```python
from build123d import *
from build123d import SkipClean  # not in build123d's __all__

# Parameters (mm, degrees)
F0_W      = 40
F0_H      = 30
F1_DEPTH  = 52
F2_R      = 5
F3_DEPTH  = 20
F4_R      = 1.65
F5_DEPTH  = 10
F6_R      = 2.5
F7_DEPTH  = 52.001
F8_R      = 4
F9_DEPTH  = 5
F10_W     = 40
F10_H     = 35
F11_DEPTH = 10
F12_W     = 40
F12_H     = 35
F13_DEPTH = 10
F15_DEPTH = 5
F16_R     = 2.15
F17_DEPTH = 40.001
F18_R     = 5
F19_DEPTH = 40.001
F20_R     = 6
F21_DEPTH = 1
F22_R     = 2.25
F23_DEPTH = 15.5358573251


with BuildPart() as f1:
    # F0 (on Top) → F1 (new body)
    with BuildSketch(Plane.XY):
        with Locations((20, 15)):
            Rectangle(F0_W, F0_H)
    extrude(amount=F1_DEPTH)

    # F2 (on face) → F3 (cut)
    with BuildSketch(Plane.XZ):
        with Locations((20, 42)):
            Circle(F2_R)
    extrude(amount=-F3_DEPTH, mode=Mode.SUBTRACT)

    # F4 (on face) → F5 (cut)
    with BuildSketch(Plane.XY.offset(52)):
        with Locations((20, 5)):
            Circle(F4_R)
        with Locations((20, 25)):
            Circle(F4_R)
    extrude(amount=-F5_DEPTH, mode=Mode.SUBTRACT)

    # F6 (on face) → F7 (cut, through all)
    with BuildSketch(Plane.XY.offset(52)):
        with Locations((5, 5)):
            Circle(F6_R)
        with Locations((5, 25)):
            Circle(F6_R)
        with Locations((35, 5)):
            Circle(F6_R)
        with Locations((35, 25)):
            Circle(F6_R)
    extrude(amount=-F7_DEPTH, mode=Mode.SUBTRACT)

    # F8 (on face) → F9 (cut)
    with BuildSketch(Plane.XY.offset(52)):
        with Locations((5, 25)):
            Circle(F8_R)
        with Locations((5, 5)):
            Circle(F8_R)
        with Locations((35, 25)):
            Circle(F8_R)
        with Locations((35, 5)):
            Circle(F8_R)
    extrude(amount=-F9_DEPTH, mode=Mode.SUBTRACT)

    # F10 (on face) → F11 (join)
    with BuildSketch(Plane.XZ):
        with Locations((20, 17.5)):
            Rectangle(F10_W, F10_H)
    extrude(amount=F11_DEPTH)

    # F12 (on face) → F13 (join)
    with BuildSketch(Plane(origin=(0, 30, 0), x_dir=(-1, 0, 0), z_dir=(0, 1, 0))):
        with Locations((-20, 17.5)):
            Rectangle(F12_W, F12_H)
    extrude(amount=F13_DEPTH)

    # F14 (on face) → F15 (cut)
    with BuildSketch(Plane.XY.offset(35)):
        with BuildLine():
            Line((6.5, 31), (33.5, 31))
            ThreePointArc((33.5, 31), (36.3284271247, 32.1715728753), (37.5, 35))
            ThreePointArc((37.5, 35), (36.3284271247, 37.8284271247), (33.5, 39))
            Line((33.5, 39), (6.5, 39))
            ThreePointArc((6.5, 39), (3.6715728753, 37.8284271247), (2.5, 35))
            ThreePointArc((2.5, 35), (3.6715728753, 32.1715728753), (6.5, 31))
        make_face()
        with BuildLine():
            Line((6.5, -9), (33.5, -9))
            ThreePointArc((33.5, -9), (36.3284271247, -7.8284271247), (37.5, -5))
            ThreePointArc((37.5, -5), (36.3284271247, -2.1715728753), (33.5, -1))
            Line((33.5, -1), (6.5, -1))
            ThreePointArc((6.5, -1), (3.6715728753, -2.1715728753), (2.5, -5))
            ThreePointArc((2.5, -5), (3.6715728753, -7.8284271247), (6.5, -9))
        make_face()
    extrude(amount=-F15_DEPTH, mode=Mode.SUBTRACT)

    # F16 (on face) → F17 (cut, through all)
    with BuildSketch(Plane(origin=(0, 0, 0), x_dir=(0, -1, 0), z_dir=(-1, 0, 0))):
        with Locations((-15, 32)):
            Circle(F16_R)
        with Locations((-35, 32)):
            Circle(F16_R)
        with Locations((5, 32)):
            Circle(F16_R)
    extrude(amount=-F17_DEPTH, mode=Mode.SUBTRACT)

    # F18 (on face) → F19 (cut, through all)
    with BuildSketch(Plane(origin=(0, 30, 0), x_dir=(-1, 0, 0), z_dir=(0, 1, 0))):
        with Locations((-20, 42)):
            Circle(F18_R)
    with SkipClean():  # cleaning this boolean's faces spoils the solid; the shape is the same uncleaned
        extrude(amount=-F19_DEPTH, mode=Mode.SUBTRACT)

    # F20 (on face) → F21 (cut)
    with BuildSketch(Plane(origin=(0, 30, 0), x_dir=(-1, 0, 0), z_dir=(0, 1, 0))):
        with Locations((-20, 42)):
            Circle(F20_R)
    with SkipClean():  # cleaning this boolean's faces spoils the solid; the shape is the same uncleaned
        extrude(amount=-F21_DEPTH, mode=Mode.SUBTRACT)

    # F22 (on face) → F23 (cut, through all)
    with BuildSketch(Plane(origin=(0, 0, 0), x_dir=(0, -1, 0), z_dir=(-1, 0, 0))):
        with Locations((-15, 42)):
            Circle(F22_R)
    with SkipClean():  # cleaning this boolean's faces spoils the solid; the shape is the same uncleaned
        extrude(amount=-F23_DEPTH, mode=Mode.SUBTRACT)


solid = f1.part
```
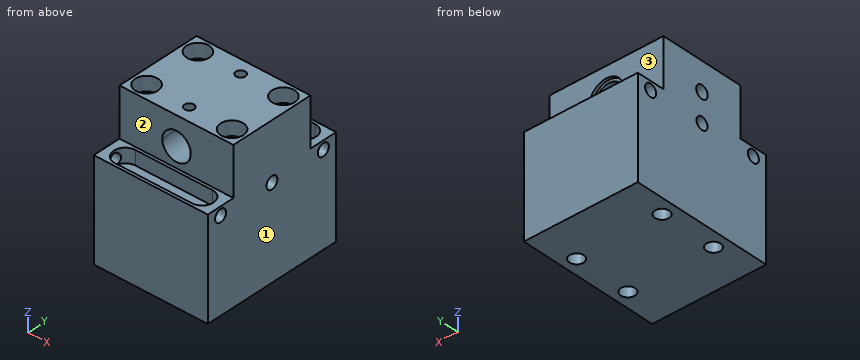
Check sheet for the modelled part. Datum: model origin and axes. Units: mm. Face numbers are marked on the shaded views. A direction names the side the tool comes from. Coordinates: 2 decimals unless noted, no trailing zeros. Write each loop counter-clockwise with the first axis right and the second up, starting at its lowest first coordinate (ties: lowest second). Pieces come first, ordered by that corner, then holes. Notation, with made-up numbers: M -34,-35.75 L 11,-35.75 A24 ccw 11,-17.75 Z; hole C 46,88.5 d6. An arc over 180 degrees is marked long. Write item = value, one per line. Start each with the question number.
1. Go/stop test with flat-tipped pins: pin 1 (5 mm diameter, centred on x = 14, y = 35.5, fed in from +Z); pin 2 (2 mm diameter, centred on x = 35.5, z = 38, fed in from +Y). Record where each tip stops, or that it passes through.
2. Sectioned sample at A-A (x = 24). State how many separate pieces and enclosed holes the cut face has, then the cut area to 3 significant figures.
3. Sectioned sample at D-D (y = 25). Record the cut outline in (x, z), then the cut area to 3 significant figures.
4. Sectioned sample at C-C (z = 18). Record the cut outline in (x, y), then the cut area to 3 significant figures.
5. Sectioned sample at B-B (y = 15). Record the cut outline in (x, z).
6. Thickness scan on probe 1 along Y at (x, z) = (5, 42); probe 2 along Y at (x, z) = (20, 48.9); probe 3 along X at (y, z) = (7, 43). Record the ranges inside material, lowest first.
7. Tool access check on the marked faces 1, 2 and 3. Record the directions out of +Z, -Z, +X, -X, +Y, -Y that give a thin tool (end or side, any length) a straight path to the whole face; none if there is none.
The answers:
q1.pin_1 = 30
q1.pin_2 = 30
q2.separate_pieces = 2
q2.enclosed_holes = 1
q2.area = 1,980 mm²
q3.outline = M 0,0 L 2.5,0 L 2.5,47 L 1,47 L 1,52 L 0,52 Z; M 7.5,0 L 32.5,0 L 32.5,47 L 31,47 L 31,52 L 21.65,52 L 21.65,46.72 A5 cw long 18.35,46.72 L 18.35,52 L 9,52 L 9,47 L 7.5,47 Z; M 37.5,0 L 40,0 L 40,52 L 39,52 L 39,47 L 37.5,47 Z
q3.area = 1,430 mm²
q4.outline = M 0,-10 L 40,-10 L 40,40 L 0,40 Z; hole C 5,5 d5; hole C 5,25 d5; hole C 35,5 d5; hole C 35,25 d5
q4.area = 1,920 mm²
q5.outline = M 0,0 L 40,0 L 40,29.85 L 0,29.85 Z; M 0,34.15 L 40,34.15 L 40,52 L 0,52 L 0,44.25 L 15.53,44.25 A5 cw long 15.53,39.75 L 0,39.75 Z
q6.probe_1 = 0 to 2.5, 7.5 to 12.75, 17.25 to 22.5, 27.5 to 30
q6.probe_2 = 0 to 3.35, 6.65 to 23.35, 26.65 to 30
q6.probe_3 = 0 to 3.5, 6.5 to 15.1, 24.9 to 33.5, 36.5 to 40
q7.face_1 = +Z, -Z, +X, +Y, -Y
q7.face_2 = +Z, +X, -X, -Y
q7.face_3 = +Z, +X, -X, +Y
